```python
from build123d import *

# Parameters (mm, degrees)
F0_W     = 0.8
F0_H     = 9
F0_W_2   = 1.2
F0_H_2   = 14.8
F1_DEPTH = 1.2
F2_DEPTH = 2
F3_DEPTH = 2
F4_DEPTH = 7.2


with BuildPart() as f1:
    # F0 (on Top) → F1 (new body)
    with BuildSketch(Plane.XY):
        Polygon((14.2, -7.4), (14.2, 7.4), (8.358179, 7.4), (5.158179, 10.4), (-5.4, 10.4), (-5.4, 4.5), (-5.4, -4.5), (-5.4, -10.4), (5.158179, -10.4), (8.358179, -7.4), align=None)
        Polygon((15.4, 8.2), (8.674537, 8.2), (5.474537, 11.2), (-6.2, 11.2), (-6.2, 4.5), (-5.4, 4.5), (-5.4, 10.4), (5.158179, 10.4), (8.358179, 7.4), (14.2, 7.4), (15.4, 7.4), align=None)
        with Locations((-5.8, 0)):
            Rectangle(F0_W, F0_H)
        Polygon((15.4, -8.2), (15.4, -7.4), (14.2, -7.4), (8.358179, -7.4), (5.158179, -10.4), (-5.4, -10.4), (-5.4, -4.5), (-6.2, -4.5), (-6.2, -11.2), (5.474537, -11.2), (8.674537, -8.2), align=None)
        with Locations((14.8, 0)):
            Rectangle(F0_W_2, F0_H_2)
    extrude(amount=F1_DEPTH)

    # F0 (on Top) → F2 (join)
    with BuildSketch(Plane.XY):
        with Locations((-5.8, 0)):
            Rectangle(F0_W, F0_H)
    extrude(amount=F2_DEPTH)

    # F0 (on Top) → F3 (join)
    with BuildSketch(Plane.XY):
        with Locations((14.8, 0)):
            Rectangle(F0_W_2, F0_H_2)
    extrude(amount=F3_DEPTH)

    # F0 (on Top) → F4 (join)
    with BuildSketch(Plane.XY):
        Polygon((15.4, 8.2), (8.674537, 8.2), (5.474537, 11.2), (-6.2, 11.2), (-6.2, 4.5), (-5.4, 4.5), (-5.4, 10.4), (5.158179, 10.4), (8.358179, 7.4), (14.2, 7.4), (15.4, 7.4), align=None)
        Polygon((15.4, -8.2), (15.4, -7.4), (14.2, -7.4), (8.358179, -7.4), (5.158179, -10.4), (-5.4, -10.4), (-5.4, -4.5), (-6.2, -4.5), (-6.2, -11.2), (5.474537, -11.2), (8.674537, -8.2), align=None)
    extrude(amount=F4_DEPTH)


solid = f1.part
```
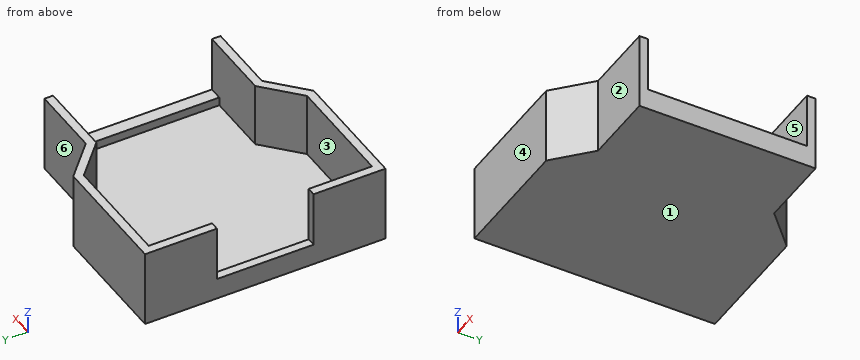
Read the model definition and answer for the solid it produces. Units are mm, in the model's axes. Face numbers are marked on the shaded views. A direction names the side the tool comes from. Round coordinates to 2 decimals unless told otherwise and drop trailing zeros. Write each loop counter-clockwise with the first axis right and the second up, starting at its lowest first coordinate (ties: lowest second). Pieces come first, ordered by that corner, then holes. Notation, with made-up numbers: M 39.5,8.25 L 65.5,8.25 A17 ccw 65.5,15.25 Z; hole C 15.25,26.5 d3. An arc over 180 degrees is marked long. One line per item, written item: value.
Q1. Find section C-C on y = 3.75. Write down the section's boundary in (x, z), plus the area to 3 significant figures.
Data:
outline: M -6.2,0 L 15.4,0 L 15.4,2 L 14.2,2 L 14.2,1.2 L -5.4,1.2 L -5.4,2 L -6.2,2 Z
area: 27.5 mm2
Q2. For a pull along Y with two mould halves and no side action, classify the marked faces 4, 5 and 6 as +Y half, -Y half, draft (parallel to the pull), parting line (faces both ways), or undercut.
Data:
face 4: -Y half
face 5: undercut
face 6: +Y half
Q3. Find section D-D on x = -0.25. Write down the section's boundary in (y, z), plus the area to 3 significant figures.
Data:
outline: M -11.2,0 L 11.2,0 L 11.2,7.2 L 10.4,7.2 L 10.4,1.2 L -10.4,1.2 L -10.4,7.2 L -11.2,7.2 Z
area: 36.5 mm2
Q4. Flat-ended cylindrical pins translate along their axes: pin 1 Ø1.5 at (x, y) = (12.5, 2.5) entering from +Z; pin 2 Ø3.5 at (x, z) = (12, 4) entering from -Y; pin 3 Ø1.8 at (x, z) = (11, 2.5) entering from +Y. Find the tip coordinate at first contact, or state that the pin passes through.
Data:
pin 1: z = 1.2
pin 2: y = -8.2
pin 3: y = 8.2
Q5. Which of the six approach directions +Z, -Z, +X, -X, +Y, -Y give full straight-line access (tool end or side, diameter ignored) to the marked faces 1, 2 and 3?
Data:
face 1: -Z, +X, -X, +Y, -Y
face 2: +Z, -Z, +X, -Y
face 3: +Z
Q6. Straight lines are drawn through the part: line 1 (Y direction, x = 9.5, z = 5.5); line 2 (Y direction, x = -4.25, z = 2.5); line 3 (Z direction, x = 9, y = -3.25). For each, find the intervals that lie inside material, in ascending order. Write a range as [from, to].
Data:
line 1: [-8.2, -7.4], [7.4, 8.2]
line 2: [-11.2, -10.4], [10.4, 11.2]
line 3: [0, 1.2]
Q7. Find section A-A on z = 1.5. Write down the section's boundary in (x, y).
Data:
outline: M -6.2,-11.2 L 5.47,-11.2 L 8.67,-8.2 L 15.4,-8.2 L 15.4,8.2 L 8.67,8.2 L 5.47,11.2 L -6.2,11.2 Z; hole M -5.4,-10.4 L 5.16,-10.4 L 8.36,-7.4 L 14.2,-7.4 L 14.2,7.4 L 8.36,7.4 L 5.16,10.4 L -5.4,10.4 Z
Q8. Find section B-B on z = 3.5. Write down the section's boundary in (x, y), plus the area to 3 significant figures.
Data:
outline: M -6.2,-11.2 L 5.47,-11.2 L 8.67,-8.2 L 15.4,-8.2 L 15.4,-7.4 L 8.36,-7.4 L 5.16,-10.4 L -5.4,-10.4 L -5.4,-4.5 L -6.2,-4.5 Z; M -6.2,4.5 L -5.4,4.5 L -5.4,10.4 L 5.16,10.4 L 8.36,7.4 L 15.4,7.4 L 15.4,8.2 L 8.67,8.2 L 5.47,11.2 L -6.2,11.2 Z
area: 45.9 mm2
